```python
from build123d import *

# Parameters (mm, degrees)
SKETCH1_W                      = 31.3
SKETCH1_H                      = 52.4
BOSS_EXTRUDE1_DEPTH            = 3
SKETCH2_W                      = 31.3
SKETCH2_H                      = 3
BOSS_EXTRUDE2_DEPTH            = 33
SKETCH3_W                      = 31.3
SKETCH3_H                      = 8.7
BOSS_EXTRUDE3_DEPTH            = 33
SKETCH5_R                      = 13.75
CUT_EXTRUDE1_DEPTH             = 8.7
SKETCH6_R                      = 6.15
CUT_EXTRUDE2_DEPTH             = 3
CUT_EXTRUDE3_REACH             = 58.546
SKETCH7_R                      = 1.7
CUT_EXTRUDE3_DIRECTION_2_REACH = 58.546
FILLET4_R                      = 0.5
CUT_EXTRUDE6_DEPTH             = 3
FILLET5_R                      = 10


with BuildPart() as part:
    # Sketch1 → Boss-Extrude1 (new body)
    with BuildSketch(Plane.XY):
        Rectangle(SKETCH1_W, SKETCH1_H)
    extrude(amount=BOSS_EXTRUDE1_DEPTH)

    # Sketch2 → Boss-Extrude2 (add)
    with BuildSketch(Plane.XY.offset(3)):
        with Locations((0, 16)):
            Rectangle(SKETCH2_W, SKETCH2_H)
    extrude(amount=BOSS_EXTRUDE2_DEPTH)

    # Sketch3 → Boss-Extrude3 (add)
    with BuildSketch(Plane.XY.offset(3)):
        with Locations((0, 21.85)):
            Rectangle(SKETCH3_W, SKETCH3_H)
    extrude(amount=BOSS_EXTRUDE3_DEPTH)

    # Sketch5 → Cut-Extrude1 (cut)
    with BuildSketch(Plane(origin=(0, 26.2, 0), x_dir=(1, 0, 0), z_dir=(0, 1, 0))):
        with Locations(Location((0, -18, 0), (0, 0, 270))):
            Circle(SKETCH5_R)
    extrude(amount=-CUT_EXTRUDE1_DEPTH, mode=Mode.SUBTRACT)

    # Sketch6 → Cut-Extrude2 (cut)
    with BuildSketch(Plane(origin=(0, 17.5, 0), x_dir=(1, 0, 0), z_dir=(0, 1, 0))):
        with Locations(Location((0, -18, 0), (0, 0, 180))):
            Circle(SKETCH6_R)
    extrude(amount=-CUT_EXTRUDE2_DEPTH, mode=Mode.SUBTRACT)

    # Cut-Extrude3: up to this face of the body (flat: up to its plane)
    cut_extrude3_end = Plane(part.part.faces().sort_by_distance((0, -26.2, 1.5))[0])
    # Sketch7 → Cut-Extrude3 (cut, up to the picked face)
    with BuildSketch(Plane.XZ.offset(-14.5), mode=Mode.PRIVATE) as cut_extrude3_sk1:
        with Locations(Location((-9, 18, 0), (0, 0, 180))):
            Circle(SKETCH7_R)
    cut_extrude3_tool1 = split(extrude(cut_extrude3_sk1.sketch, amount=CUT_EXTRUDE3_REACH, mode=Mode.PRIVATE), bisect_by=cut_extrude3_end, keep=Keep.BOTH, mode=Mode.PRIVATE)
    # Sketch7 → Cut-Extrude3 (cut, up to the picked face)
    with BuildSketch(Plane.XZ.offset(-14.5), mode=Mode.PRIVATE) as cut_extrude3_sk2:
        with Locations(Location((9, 18, 0), (0, 0, 180))):
            Circle(SKETCH7_R)
    cut_extrude3_tool2 = split(extrude(cut_extrude3_sk2.sketch, amount=CUT_EXTRUDE3_REACH, mode=Mode.PRIVATE), bisect_by=cut_extrude3_end, keep=Keep.BOTH, mode=Mode.PRIVATE)
    add(cut_extrude3_tool1.solids().sort_by(Axis((-9, 14.5, 18), (0, -1, 0)))[0], mode=Mode.SUBTRACT)
    add(cut_extrude3_tool2.solids().sort_by(Axis((9, 14.5, 18), (0, -1, 0)))[0], mode=Mode.SUBTRACT)

    # Cut-Extrude3 direction 2: up to this face of the body (flat: up to its plane)
    cut_extrude3_direction_2_end = Plane(part.part.faces().sort_by_distance((0, 17.5, 4.63890873))[0])
    # Sketch7 → Cut-Extrude3 direction 2 (cut, up to the picked face)
    with BuildSketch(Plane.XZ.offset(-14.5), mode=Mode.PRIVATE) as cut_extrude3_direction_2_sk1:
        with Locations(Location((-9, 18, 0), (0, 0, 180))):
            Circle(SKETCH7_R)
    cut_extrude3_direction_2_tool1 = split(extrude(cut_extrude3_direction_2_sk1.sketch, amount=-CUT_EXTRUDE3_DIRECTION_2_REACH, mode=Mode.PRIVATE), bisect_by=cut_extrude3_direction_2_end, keep=Keep.BOTH, mode=Mode.PRIVATE)
    # Sketch7 → Cut-Extrude3 direction 2 (cut, up to the picked face)
    with BuildSketch(Plane.XZ.offset(-14.5), mode=Mode.PRIVATE) as cut_extrude3_direction_2_sk2:
        with Locations(Location((9, 18, 0), (0, 0, 180))):
            Circle(SKETCH7_R)
    cut_extrude3_direction_2_tool2 = split(extrude(cut_extrude3_direction_2_sk2.sketch, amount=-CUT_EXTRUDE3_DIRECTION_2_REACH, mode=Mode.PRIVATE), bisect_by=cut_extrude3_direction_2_end, keep=Keep.BOTH, mode=Mode.PRIVATE)
    add(cut_extrude3_direction_2_tool1.solids().sort_by(Axis((-9, 14.5, 18), (0, 1, 0)))[0], mode=Mode.SUBTRACT)
    add(cut_extrude3_direction_2_tool2.solids().sort_by(Axis((9, 14.5, 18), (0, 1, 0)))[0], mode=Mode.SUBTRACT)

    # Fillet4
    fillet4_edges = [part.edges().sort_by_distance(p)[0] for p in [
        (0, 17.5, 4.25),
        (6.15, 17.5, 18),
        (-7.3, 17.5, 18),
        (10.7, 17.5, 18),
    ]]
    fillet(fillet4_edges, radius=FILLET4_R)

    # Sketch10 → Cut-Extrude6 (cut)
    with BuildSketch(Plane(origin=(0, 0, 0), x_dir=(-1, 0, 0), z_dir=(0, 0, -1))):
        with BuildLine():
            Line((-2.55, -11.5), (-2.55, -8.5))
            ThreePointArc((-2.55, -8.5), (0, -5.95), (2.55, -8.5))
            Line((2.55, -8.5), (2.55, -11.5))
            ThreePointArc((2.55, -11.5), (0, -14.05), (-2.55, -11.5))
        make_face()
        with BuildLine():
            Line((-2.55, 8.5), (-2.55, 11.5))
            ThreePointArc((-2.55, 11.5), (0, 14.05), (2.55, 11.5))
            Line((2.55, 11.5), (2.55, 8.5))
            ThreePointArc((2.55, 8.5), (0, 5.95), (-2.55, 8.5))
        make_face()
    extrude(amount=-CUT_EXTRUDE6_DEPTH, mode=Mode.SUBTRACT)

    # Fillet5
    fillet5_edges = [part.edges().sort_by_distance(p)[0] for p in [
        (15.65, -26.2, 1.5),
        (-15.65, -26.2, 1.5),
    ]]
    fillet(fillet5_edges, radius=FILLET5_R)


solid = part.part
```
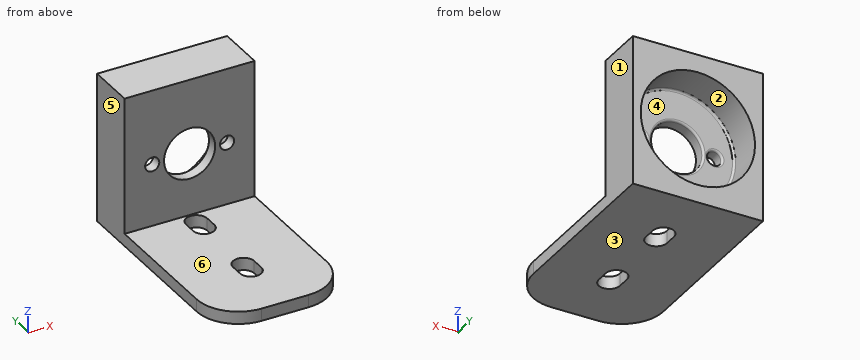
Part model, mm, in its own coordinate system. Face numbers are marked on the shaded views. A direction names the side the tool comes from. Round coordinates to 2 decimals unless told otherwise and drop trailing zeros. Write each loop counter-clockwise with the first axis right and the second up, starting at its lowest first coordinate (ties: lowest second). Pieces come first, ordered by that corner, then holes. Notation, with made-up numbers: (-37.5, -20) -> (-8.5, -20) arc R20 ccw to (-8.5, -5) -> close; hole circle Ø8 at (14, 27). An arc over 180 degrees is marked (long way). Return JSON: item names as keys, results as strings. Group by question number.
Q1. Probe L1, parallel to Z at x = 12.5, y = -16; L2, parallel to Z at x = 0, y = 15.3; L3, parallel to Y at x = -10, z = 30. List the from-to ranges inside material, lowest first. Write a range as [from, to].
Q2. Saw through at A-A on x = 0. Write the cut outline in (y, z), plus the area to 3 significant figures.
Q3. Mould opens along Z. For the marked faces 1, 2, 3 and 4 say: pulls with the +Z half, pulls with the -Z half, needs draft (parallel to the pull), parting line crosses it, or undercut.
Q4. Pin check, flat tips, straight feed: pin 1 (4 mm diameter, centred on x = 9, z = 18, fed in from +Y); pin 2 (4 mm diameter, centred on x = 9, y = -10, fed in from +Z); pin 3 (6 mm diameter, centred on x = 12.5, z = 29.5, fed in from -Y). Stop position of each tip, or through.
Q5. Saw through at B-B on y = -3.5. Write the cut outline in (x, z).
Q6. Saw through at C-C on y = -20. Write the cut outline in (x, z), plus the area to 3 significant figures.
Q7. Which spindle directions (+Z, -Z, +X, -X, +Y, -Y) get a long thin tool onto all of the face, cutting with end or side? Do the marked faces 5 and 6. Say none if no direction does.
Answer:
{
 "1": {"L1": "[0, 3]", "L2": "[0, 11.85], [24.15, 36]", "L3": "[14.5, 26.2]"},
 "2": {"outline": "(-26.2, 0) -> (-14.05, 0) -> (-14.05, 3) -> (-26.2, 3) -> close; (-5.95, 0) -> (5.95, 0) -> (5.95, 3) -> (-5.95, 3) -> close; (14.05, 0) -> (26.2, 0) -> (26.2, 4.25) -> (18, 4.25) arc R0.5 cw to (17.5, 4.75) -> (17.5, 11.35) arc R0.5 ccw to (17, 11.85) -> (14.5, 11.85) -> (14.5, 3) -> (14.05, 3) -> close; (14.5, 24.15) -> (17, 24.15) arc R0.5 ccw to (17.5, 24.65) -> (17.5, 31.25) arc R0.5 cw to (18, 31.75) -> (26.2, 31.75) -> (26.2, 36) -> (14.5, 36) -> close", "area": "219 mm2"},
 "3": {"face 1": "needs draft", "face 2": "undercut", "face 3": "pulls with the -Z half", "face 4": "undercut"},
 "4": {"pin 1": "y = 17.46", "pin 2": "z = 3", "pin 3": "y = 14.5"},
 "5": {"outline": "(-15.65, 0) -> (15.65, 0) -> (15.65, 3) -> (-15.65, 3) -> close"},
 "6": {"outline": "(-14.9, 0) -> (14.9, 0) -> (14.9, 3) -> (-14.9, 3) -> close", "area": "89.4 mm2"},
 "7": {"face 5": "+Z, -Z, -X, +Y, -Y", "face 6": "+Z, +X, -X, -Y"}
}
